Part model, mm, in its own coordinate system. A direction names the side the tool comes from. Give positions to 0.01 mm unless a question says otherwise; leave off trailing zeros. Order: outer loops, then holes, each group sorted by start corner. A loop starts at its lowest first (then second) coordinate and runs counter-clockwise, first axis right, second up. Notation, with made-up numbers: (22.25, -28.75) - (79.25, -28.75) arc R26 ccw to (79.25, -2.75) - close; hole circle Ø5 at (-3, -23). An arc over 180 degrees is marked (long way). Use one line per item in the form item = value. Start each with the question number.
1. Band-saw the part on C-C, the plane z = 8. List the corners of the cut face in (x, y), plus the area to 3 significant figures.
2. Band-saw the part on D-D, the plane x = 4.25. List the corners of the cut face in (y, z).
3. Band-saw the part on B-B, the plane x = 1.5. List the corners of the cut face in (y, z) (3 decimals).
4. Band-saw the part on A-A, the plane y = -3. List the corners of the cut face in (x, z), plus the area to 3 significant figures.
5. Tool access for faces 1 (the face through (13, 0, 0)), 2 (the face through (2, 6.35, 21)), 3 (the face through (15.24, 0, 10)): list every direction of +Z, -Z, +X, -X, +Y, -Y with a clear straight run to the whole face (end or side of a thin tool).
6. Drill centre lines: line 1 (Y direction, x = 18.5, z = 6.75); line 2 (Z direction, x = 23, y = -14); line 3 (Y direction, x = 5.75, z = 6.5). Where is each one in solid material? Low to high.
7. Pin check, flat tips, straight feed: P1, Ø2.5, axis at y = 1.5, z = 11.5, coming from the +X side; P2, Ø4, axis at x = 5, y = 0.5, coming from the +Z side; P3, Ø6.5, axis at x = 11, z = 14.5, coming from the -Y side. Stop position of each tip, or through.
from build123d import *

# Parameters (mm, degrees)
F0_W     = 25.4
F0_H     = 6.35
F1_DEPTH = 19.05
F3_DEPTH = 12.7
F4_W     = 12.7
F4_H     = 12.7
F5_DEPTH = 15.24
F6_DEPTH = 25.4


with BuildPart() as f1:
    # F0 (on Front) → F1 (new body, symmetric)
    with BuildSketch(Plane.XZ):
        with Locations((12.7, 3.175)):
            Rectangle(F0_W, F0_H)
    extrude(amount=F1_DEPTH, both=True)

    # F2 (on face) → F3 (join)
    with BuildSketch(Plane(origin=(0, 19.05, 0), x_dir=(-1, 0, 0), z_dir=(0, 1, 0))):
        Polygon((-25.4, 6.35), (0, 6.35), (0, 25.4), align=None)
    extrude(amount=-F3_DEPTH)

    # F4 (on face) → F5 (join)
    with BuildSketch(Plane(origin=(0, 0, 0), x_dir=(0, -1, 0), z_dir=(-1, 0, 0))):
        with Locations((0, 12.7)):
            Rectangle(F4_W, F4_H)
    extrude(amount=-F5_DEPTH)

    # F6 (cut): a face of the model
    f6_faces = [f1.faces().sort_by_distance(p)[0] for p in [
        (12.9822222222, 6.35, 17.3566666667),
    ]]
    extrude(f6_faces, amount=-F6_DEPTH, mode=Mode.SUBTRACT)


solid = f1.part
From the geometry:
q1.outline = (0, -6.35) - (15.24, -6.35) - (15.24, 6.35) - (23.2, 6.35) - (23.2, 19.05) - (0, 19.05) - close
q1.area = 488 mm²
q2.outline = (-19.05, 0) - (19.05, 0) - (19.05, 22.21) - (6.35, 22.21) - (6.35, 19.05) - (-6.35, 19.05) - (-6.35, 6.35) - (-19.05, 6.35) - close
q3.outline = (-19.05, 0) - (19.05, 0) - (19.05, 24.275) - (6.35, 24.275) - (6.35, 19.05) - (-6.35, 19.05) - (-6.35, 6.35) - (-19.05, 6.35) - close
q4.outline = (0, 0) - (25.4, 0) - (25.4, 6.35) - (15.24, 6.35) - (15.24, 13.97) - (8.47, 19.05) - (0, 19.05) - close
q4.area = 338 mm²
q5.face_1 = -Z, +X, -X, +Y, -Y
q5.face_2 = +Z, +X, -X, -Y
q5.face_3 = +Z, +X, -Y
q6.line_1 = 6.35 to 19.05
q6.line_2 = 0 to 6.35
q6.line_3 = -6.35 to 19.05
q7.P1 = 15.24
q7.P2 = 19.05
q7.P3 = -6.35
